The figure shows three views and two pictorial views of one solid part (mm, origin at its lowest corner). Answer the questions. Round coordinates to 2 decimals unless told otherwise and drop trailing zeros. Write each loop counter-clockwise with the first axis right and the second up, starting at its lowest first coordinate (ties: lowest second). Pieces come first, ordered by that corner, then holes. Notation, with made-up numbers: (65.25, 27) - (92.25, 27) arc R31 cw to (92.25, 54) - close; hole circle Ø7 at (55, 3). An arc over 180 degrees is marked (long way). Answer as CSV lines item,"result". Start each with the question number.
Item 1: A cutting plane is placed at D-D on y = 17.5. Determine the outline of the cut face in (x, z) (1 decimal).
Item 2: A flat-ended cylindrical pin translates along its axis: pin 1 (1.5 mm diameter, centred on x = 3, y = 18, fed in from +Z). Find the tip coordinate at first contact, or state that the pin passes through.
Item 3: A cutting plane is placed at A-A on x = 3.75. State how many separate pieces and enclosed holes the cut face has.
Item 4: Straight lines are drawn through the part: line 1 along Y through (x, z) = (3.25, 0.3) (1 decimal); line 2 along Y through (x, z) = (3, 0.6) (1 decimal); line 3 along X through (y, z) = (11.5, 0.2). For each, find the intervals that lie inside material, in ascending order. Write a range as [from, to].
Item 5: A cutting plane is placed at B-B on y = 2.5. Determine the outline of the cut face in (x, z).
Item 6: For a pull along X with two mould halves and no side action, classify the marked faces 1, 2, 3 and 4 as pulls with the +X half, pulls with the -X half, needs draft (parallel to the pull), parting line crosses it, or undercut.
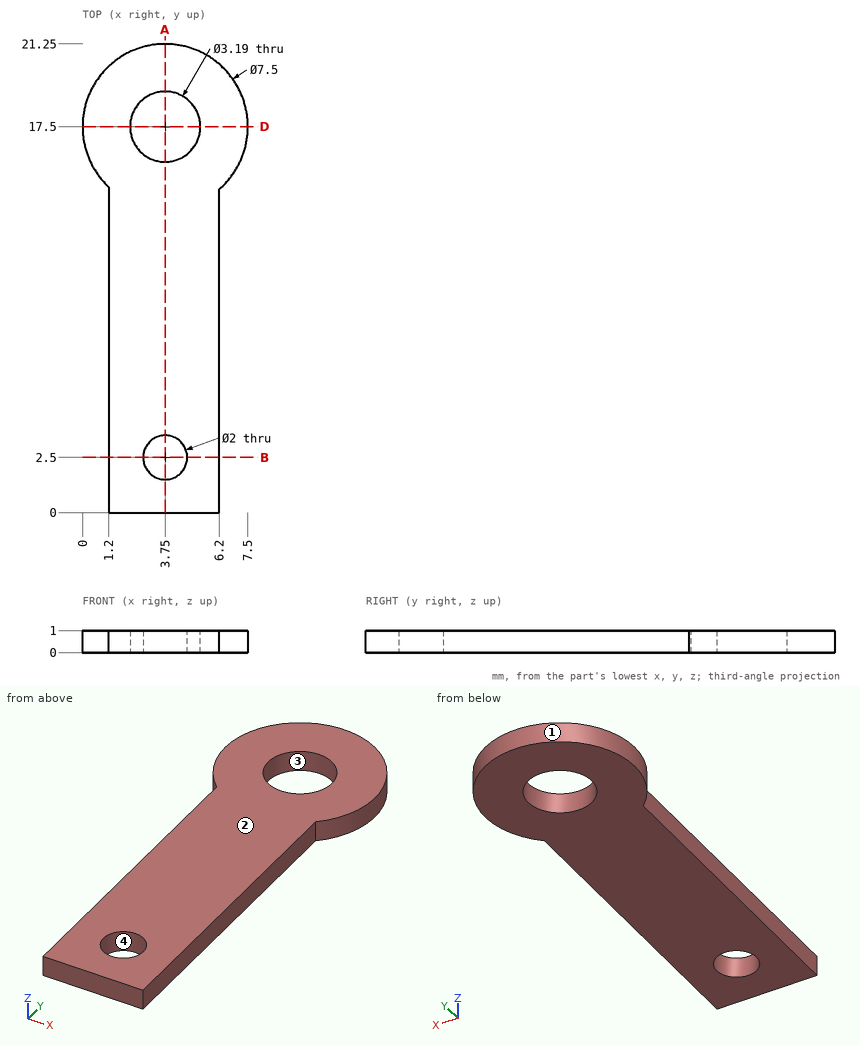
Geometry says:
1,outline,"(0, 0) - (2.2, 0) - (2.2, 1) - (0, 1) - close; (5.3, 0) - (7.5, 0) - (7.5, 1) - (5.3, 1) - close"
2,pin 1,"stops at z = 1"
3,separate pieces,"3"
3,enclosed holes,"0"
4,line 1,"y = [0, 1.6], [3.4, 16], [19, 21.2]"
4,line 2,"y = [0, 1.8], [3.2, 16.1], [18.9, 21.2]"
4,line 3,"x = [1.2, 6.2]"
5,outline,"(1.2, 0) - (2.75, 0) - (2.75, 1) - (1.2, 1) - close; (4.75, 0) - (6.2, 0) - (6.2, 1) - (4.75, 1) - close"
6,face 1,"parting line crosses it"
6,face 2,"needs draft"
6,face 3,"undercut"
6,face 4,"undercut"
